Geometry: final body of the model. Coordinates: model frame, mm. Face numbers are marked on the shaded views. A direction names the side the tool comes from. Coordinates: 2 decimals unless noted, no trailing zeros. Order: outer loops, then holes, each group sorted by start corner. A loop starts at its lowest first (then second) coordinate and runs counter-clockwise, first axis right, second up. Notation, with made-up numbers: (6, -26) -> (14, -26) arc R24 cw to (14, -4) -> close; hole circle Ø2 at (-14, 84.5). An arc over 180 degrees is marked (long way). Use CSV: the item, a comma, the result in double quotes. Start each with the question number.
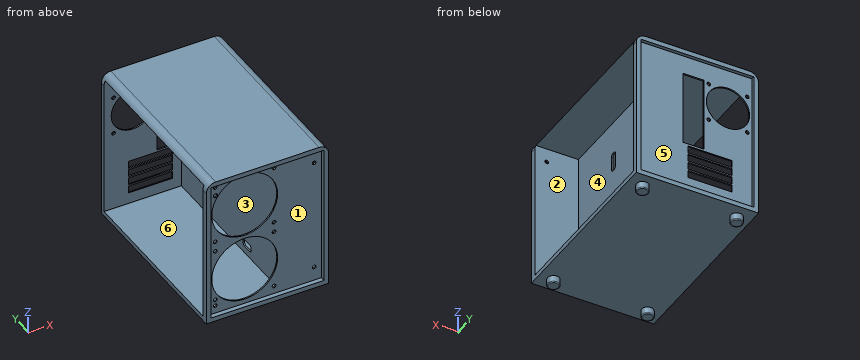
from build123d import *

# Parameters (mm, degrees)
F0_W         = 260
F0_H         = 397
F1_DEPTH     = 320
F2_W         = 240
F2_H         = 300
F3_DEPTH     = 506.73
F5_DEPTH     = 304.8
F6_W         = 3
F6_H         = 377
F7_DEPTH     = 300
F8_R         = 12.5
F9_DEPTH     = 15
F10_R        = 2
F11_W        = 3
F11_H        = 377
F12_DEPTH    = 300
F13_W        = 3
F13_H        = 300
F14_DEPTH    = 87
F15_W        = 3
F15_H        = 300
F16_DEPTH    = 160
F17_R        = 4
F17_R_2      = 70
F18_DEPTH    = 10
F19_W        = 344
F19_H        = 300
F20_DEPTH    = 206
F21_W        = 240
F21_H        = 3
F22_DEPTH    = 300
F23_W        = 44
F23_H        = 159
F23_W_2      = 93.7
F23_H_2      = 15.9
F24_DEPTH    = 25
F25_R        = 4
F25_R_2      = 46
F26_DEPTH    = 25
F27_W        = 3
F27_H        = 300
F28_DEPTH    = 377
F29_W        = 30
F29_H        = 300
F30_DEPTH    = 25
F31_W        = 161.3201568723
F31_H        = 300
F32_DEPTH    = 25
F33_W        = 164.3201568723
F33_H        = 3
F34_DEPTH    = 300
F35_T1_DEPTH = 497
F36_R        = 70
F36_R_2      = 4
F37_DEPTH    = 25
F38_W        = 377
F38_H        = 300
F39_DEPTH    = 3
F40_W        = 5.6798431277
F40_H        = 300
F41_DEPTH    = 3
F42_T1_DEPTH = 497
F43_W        = 3
F43_H        = 374
F44_DEPTH    = 300
F45_W        = 3
F45_H        = 374
F46_DEPTH    = 300
F47_W        = 25
F47_H        = 15
F48_DEPTH    = 25
F49_R        = 5
F51_W        = 15
F51_H        = 40
F51_W_2      = 30
F51_H_2      = 15
F52_DEPTH    = 25
F53_R        = 5
F54_R        = 5
F56_DEPTH    = 25


# Not quite as in the source:
# - a fillet or chamfer that OpenCascade refuses, or shapes differently, is made with other operations: its cross-section is extruded or revolved along the edge and cut away or added


with BuildPart() as f1:
    # F0 (on Top) → F1 (new body)
    with BuildSketch(Plane.XY):
        Rectangle(F0_W, F0_H)
    extrude(amount=F1_DEPTH)

    # F2 (on face) → F3 (cut)
    with BuildSketch(Plane.XZ.offset(198.5)):
        with Locations((0, 160)):
            Rectangle(F2_W, F2_H)
    extrude(amount=-F3_DEPTH, mode=Mode.SUBTRACT)

    # F4 (on face) → F5 (cut)
    with BuildSketch(Plane(origin=(-130, 0, 0), x_dir=(0, -1, 0), z_dir=(-1, 0, 0))):
        Polygon((188.5, 10), (188.5, 310), (-188.5, 310), (-188.5, 10), (0, 10), align=None)
    extrude(amount=-F5_DEPTH, mode=Mode.SUBTRACT)

    # F6 (on face) → F7 (join)
    with BuildSketch(Plane.XY.offset(10)):
        with Locations((-125.8077577353, 0)):
            Rectangle(F6_W, F6_H)
        with Locations((125.8201568723, 0)):
            Rectangle(F6_W, F6_H)
    extrude(amount=F7_DEPTH)

    # F8 (on face) → F9 (join)
    with BuildSketch(Plane(origin=(0, 0, 0), x_dir=(1, 0, 0), z_dir=(0, 0, -1))):
        with Locations((-100, 168.5)):
            Circle(F8_R)
        with Locations((100, 168.5)):
            Circle(F8_R)
        with Locations((100, -168.5)):
            Circle(F8_R)
        with Locations((-100, -168.5)):
            Circle(F8_R)
    extrude(amount=F9_DEPTH)

    # F10
    f10_edges = [f1.edges().sort_by_distance(p)[0] for p in [
        (-112.5, -168.5, -15),
        (87.5, -168.5, -15),
        (87.5, 168.5, -15),
        (-112.5, 168.5, -15),
    ]]
    fillet(f10_edges, radius=F10_R)

    # F11 (on face) → F12 (join)
    with BuildSketch(Plane.XY.offset(10)):
        with Locations((35.8201568723, 0)):
            Rectangle(F11_W, F11_H)
    extrude(amount=F12_DEPTH)

    # F13 (on face) → F14 (join)
    with BuildSketch(Plane.YZ.offset(37.3201568723)):
        with Locations((-187, 160)):
            Rectangle(F13_W, F13_H)
    extrude(amount=F14_DEPTH)

    # F15 (on face) → F16 (join)
    with BuildSketch(Plane(origin=(34.3201568723, 0, 0), x_dir=(0, -1, 0), z_dir=(-1, 0, 0))):
        with Locations((157, 160)):
            Rectangle(F15_W, F15_H)
    extrude(amount=F16_DEPTH)

    # F17 (on face) → F18 (cut)
    with BuildSketch(Plane.XZ.offset(158.5)):
        with Locations((-105.3498431277, 299)):
            Circle(F17_R)
        with Locations((19.6501568723, 299)):
            Circle(F17_R)
        with Locations((-105.3498431277, 174)):
            Circle(F17_R)
        with Locations((19.6501568723, 174)):
            Circle(F17_R)
        with Locations((-42.8498431277, 236.5)):
            Circle(F17_R_2)
        with Locations((-42.8498431277, 83.5)):
            Circle(F17_R_2)
        with Locations((19.6501568723, 146)):
            Circle(F17_R)
        with Locations((19.6501568723, 21)):
            Circle(F17_R)
        with Locations((-105.3498431277, 21)):
            Circle(F17_R)
        with Locations((-105.3498431277, 146)):
            Circle(F17_R)
    extrude(amount=-F18_DEPTH, mode=Mode.SUBTRACT)

    # F19 (on face) → F20 (cut)
    with BuildSketch(Plane.YZ.offset(-124.3077577353)):
        with Locations((16.5, 160)):
            Rectangle(F19_W, F19_H)
    extrude(amount=-F20_DEPTH, mode=Mode.SUBTRACT)

    # F21 (on face) → F22 (join)
    with BuildSketch(Plane.XY.offset(10)):
        with Locations((0, 190)):
            Rectangle(F21_W, F21_H)
    extrude(amount=F22_DEPTH)

    # F23 (on face) → F24 (cut)
    with BuildSketch(Plane.XZ.offset(-188.5)):
        with Locations((4.3201568723, 190.5)):
            Rectangle(F23_W, F23_H)
        with Locations((-30.9022790795, 79.7601031285)):
            Rectangle(F23_W_2, F23_H_2)
        with Locations((-30.8398431277, 98.66)):
            Rectangle(F23_W_2, F23_H_2)
        with Locations((-30.9647150313, 60.8602062571)):
            Rectangle(F23_W_2, F23_H_2)
        with Locations((-31.0271509831, 41.9603093856)):
            Rectangle(F23_W_2, F23_H_2)
    extrude(amount=-F24_DEPTH, mode=Mode.SUBTRACT)

    # F25 (on face) → F26 (cut)
    with BuildSketch(Plane(origin=(0, 191.5, 0), x_dir=(-1, 0, 0), z_dir=(0, 1, 0))):
        with Locations((27.8399215639, 265)):
            Circle(F25_R)
        with Locations((109.8399215639, 265)):
            Circle(F25_R)
        with Locations((27.8399215639, 183)):
            Circle(F25_R)
        with Locations((109.8399215639, 183)):
            Circle(F25_R)
        with Locations((68.8399215639, 224)):
            Circle(F25_R_2)
    extrude(amount=-F26_DEPTH, mode=Mode.SUBTRACT)

    # F27 (on face) → F28 (cut)
    with BuildSketch(Plane.XZ.offset(-188.5)):
        with Locations((-128.5, 160)):
            Rectangle(F27_W, F27_H)
    extrude(amount=F28_DEPTH, mode=Mode.SUBTRACT)

    # F29 (on face) → F30 (cut)
    with BuildSketch(Plane(origin=(-127, 0, 0), x_dir=(0, -1, 0), z_dir=(-1, 0, 0))):
        with Locations((173.5, 160)):
            Rectangle(F29_W, F29_H)
    extrude(amount=-F30_DEPTH, mode=Mode.SUBTRACT)

    # F31 (on face) → F32 (cut)
    with BuildSketch(Plane(origin=(0, -155.5, 0), x_dir=(-1, 0, 0), z_dir=(0, 1, 0))):
        with Locations((46.3399215639, 160)):
            Rectangle(F31_W, F31_H)
    extrude(amount=-F32_DEPTH, mode=Mode.SUBTRACT)

    # F33 (on face) → F34 (join)
    with BuildSketch(Plane.XY.offset(10)):
        with Locations((-47.8399215639, -187)):
            Rectangle(F33_W, F33_H)
    extrude(amount=F34_DEPTH)

    # F35: fillet of radius 20 on 1 edges, made by hand

    # F35_s2 → F35_t1 (cut)
    with BuildSketch(Plane.XZ.offset(-248.5)):
        with BuildLine():
            ThreePointArc((-130, 300), (-124.1421356237, 314.1421356237), (-110, 320))
            Line((-110, 320), (-130, 320))
            Line((-130, 320), (-130, 300))
        make_face()
    extrude(amount=F35_T1_DEPTH, mode=Mode.SUBTRACT)

    # F36 (on face) → F37 (cut)
    with BuildSketch(Plane.XZ.offset(188.5)):
        with Locations((-42.84, 236.5)):
            Circle(F36_R)
        with Locations((-105.34, 299)):
            Circle(F36_R_2)
        with Locations((19.66, 299)):
            Circle(F36_R_2)
        with Locations((-105.34, 174)):
            Circle(F36_R_2)
        with Locations((19.66, 174)):
            Circle(F36_R_2)
        with Locations((-42.84, 89.5)):
            Circle(F36_R)
        with Locations((-105.34, 152)):
            Circle(F36_R_2)
        with Locations((19.66, 152)):
            Circle(F36_R_2)
        with Locations((19.66, 27)):
            Circle(F36_R_2)
        with Locations((-105.34, 27)):
            Circle(F36_R_2)
    extrude(amount=-F37_DEPTH, mode=Mode.SUBTRACT)

    # F38 (on face) → F39 (cut)
    with BuildSketch(Plane.YZ.offset(127.3201568723)):
        with Locations((0, 160)):
            Rectangle(F38_W, F38_H)
    extrude(amount=-F39_DEPTH, mode=Mode.SUBTRACT)

    # F40 (on face) → F41 (join)
    with BuildSketch(Plane(origin=(0, -188.5, 0), x_dir=(-1, 0, 0), z_dir=(0, 1, 0))):
        with Locations((-127.1600784361, 160)):
            Rectangle(F40_W, F40_H)
    extrude(amount=F41_DEPTH)

    # F42: fillet of radius 20 on 1 edges, made by hand

    # F42_s2 → F42_t1 (cut)
    with BuildSketch(Plane.XZ.offset(-248.5)):
        with BuildLine():
            ThreePointArc((110, 320), (124.1421356237, 314.1421356237), (130, 300))
            Line((130, 300), (130, 320))
            Line((130, 320), (110, 320))
        make_face()
    extrude(amount=F42_T1_DEPTH, mode=Mode.SUBTRACT)

    # F47 (on face) → F48 (cut)
    with BuildSketch(Plane(origin=(34.3201568723, 0, 0), x_dir=(0, -1, 0), z_dir=(-1, 0, 0))):
        with Locations((-148.5, 280)):
            Rectangle(F47_W, F47_H)
    extrude(amount=-F48_DEPTH, mode=Mode.SUBTRACT)

    # F49
    f49_edges = [f1.edges().sort_by_distance(p)[0] for p in [
        (35.820157, 161, 272.5),
        (35.820157, 161, 287.5),
        (35.820157, 136, 287.5),
        (35.820157, 136, 272.5),
    ]]
    fillet(f49_edges, radius=F49_R)

    # F51 (on face) → F52 (cut)
    with BuildSketch(Plane.YZ.offset(37.3201568723)):
        with Locations((-53, 220.0625501573)):
            Rectangle(F51_W, F51_H)
        with Locations((-60.5, 32.5625501573)):
            Rectangle(F51_W_2, F51_H_2)
    extrude(amount=-F52_DEPTH, mode=Mode.SUBTRACT)

    # F53
    f53_edges = [f1.edges().sort_by_distance(p)[0] for p in [
        (35.820157, -75.5, 25.06255),
        (35.820157, -75.5, 40.06255),
        (35.820157, -45.5, 25.06255),
        (35.820157, -45.5, 40.06255),
    ]]
    fillet(f53_edges, radius=F53_R)

    # F54
    f54_edges = [f1.edges().sort_by_distance(p)[0] for p in [
        (35.820157, -60.5, 200.06255),
        (35.820157, -45.5, 200.06255),
        (35.820157, -45.5, 240.06255),
        (35.820157, -60.5, 240.06255),
    ]]
    fillet(f54_edges, radius=F54_R)

    # F55 (on face) → F56 (cut)
    with BuildSketch(Plane.XZ.offset(198.5)):
        with BuildLine():
            ThreePointArc((-101, 40), (-105, 44), (-109, 40))
            Line((-109, 40), (-105, 40))
            Line((-105, 40), (-105, 36))
            ThreePointArc((-105, 36), (-102.1715728753, 37.1715728753), (-101, 40))
        make_face()
        with BuildLine():
            Line((-105, 40), (-109, 40))
            ThreePointArc((-109, 40), (-107.8284271247, 37.1715728753), (-105, 36))
            Line((-105, 36), (-105, 40))
        make_face()
        with BuildLine():
            ThreePointArc((105, 36), (107.8284271247, 37.1715728753), (109, 40))
            Line((109, 40), (105, 40))
            Line((105, 40), (105, 36))
        make_face()
        with BuildLine():
            Line((105, 40), (109, 40))
            ThreePointArc((109, 40), (102.1715728753, 42.8284271247), (105, 36))
            Line((105, 36), (105, 40))
        make_face()
        with BuildLine():
            ThreePointArc((105, 284), (102.1715728753, 277.1715728753), (109, 280))
            Line((109, 280), (105, 280))
            Line((105, 280), (105, 284))
        make_face()
        with BuildLine():
            Line((105, 280), (109, 280))
            ThreePointArc((109, 280), (107.8284271247, 282.8284271247), (105, 284))
            Line((105, 284), (105, 280))
        make_face()
        with BuildLine():
            ThreePointArc((-105, 284.5), (-108.1819805153, 283.1819805153), (-109.5, 280))
            Line((-109.5, 280), (-105, 280))
            Line((-105, 280), (-105, 284.5))
        make_face()
        with BuildLine():
            Line((-105, 280), (-109.5, 280))
            ThreePointArc((-109.5, 280), (-105, 275.5), (-100.5, 280))
            ThreePointArc((-100.5, 280), (-101.8180194847, 283.1819805153), (-105, 284.5))
            Line((-105, 284.5), (-105, 280))
        make_face()
    extrude(amount=-F56_DEPTH, mode=Mode.SUBTRACT)


with BuildPart() as f44:
    # F43 (on face) → F44 (new body)
    with BuildSketch(Plane(origin=(0, 0, 310), x_dir=(1, 0, 0), z_dir=(0, 0, -1))):
        with Locations((-125.8205080757, -1.5)):
            Rectangle(F43_W, F43_H)
    extrude(amount=F44_DEPTH)


with BuildPart() as f46:
    # F45 (on face) → F46 (new body)
    with BuildSketch(Plane(origin=(0, 0, 310), x_dir=(1, 0, 0), z_dir=(0, 0, -1))):
        with Locations((125.8205080757, -1.5)):
            Rectangle(F45_W, F45_H)
    extrude(amount=F46_DEPTH)


solid = f1.part
(1) Access query for the marked faces 4, 5 and 6. Directions: +Z, -Z, +X, -X, +Y, -Y. A direction counts if a zero-diameter tool reaches every point of the face in a straight line with its end or side. Return the directions, or none.
(2) First-contact query: pin 1 (13 mm diameter, centred on x = -27.84, z = 183, fed in from +Y); pin 2 (8 mm diameter, centred on x = 100, y = 102, fed in from -Z); pin 3 (6.5 mm diameter, centred on x = 105, z = 40, fed in from -Y). Flat tips, straight axial feed; report the tip coordinate or a pass-through.
(3) Line query: line 1 (Z direction, x = 105, y = -186); line 2 (Y direction, x = -115, z = 181); line 3 (Z direction, x = 1, y = -120). Output: solid intervals per line, ascending. Write a range as from..to.
(4) Section B-B (x = -42.84). State how many separate pieces and enclosed holes the cut face has, then the cut area to 3 significant figures.
(5) Section A-A (y = 57). Return loops of the section in (x, z).
(6) Mould query, pull axis X, two halves, no side actions, for the marked faces 1, 2 and 3. Classes: pulls with the +X half, pulls with the -X half, needs draft (parallel to the pull), parting line crosses it, or undercut.
Check sheet entries:
1,face 4,"+X"
1,face 5,"+Y"
1,face 6,"-X"
2,pin 1,"stops at y = 191.5"
2,pin 2,"stops at z = 0"
2,pin 3,"stops at y = 188.5"
3,line 1,"z = 0..36, 44..276, 284..320"
3,line 2,"y = -188.5..-185.5, 188.5..191.5"
3,line 3,"z = 0..10, 310..320"
4,separate pieces,"7"
4,enclosed holes,"0"
4,area,"8,480 mm^2"
5,outline,"(-130, 0) -> (130, 0) -> (130, 10) -> (37.32, 10) -> (37.32, 310) -> (127.32, 310) arc R20 ccw to (110, 320) -> (-110, 320) arc R20 ccw to (-127.32, 310) -> (34.32, 310) -> (34.32, 10) -> (-130, 10) -> close"
6,face 1,"undercut"
6,face 2,"needs draft"
6,face 3,"pulls with the -X half"
